from build123d import *

# Parameters (mm, degrees)
BOSS_EXTRUDE1_DEPTH = 3.175


with BuildPart() as part:
    # Sketch1 → Boss-Extrude1 (new body)
    with BuildSketch(Plane.XY):
        with BuildLine():
            Line((0, 0), (0, -1.8034))
            Line((0, -1.8034), (1.778, -6.8834))
            Line((1.778, -6.8834), (1.778, -23.3934))
            Line((1.778, -23.3934), (0, -28.4734))
            Line((0, -28.4734), (0, -33.02))
            Line((0, -33.02), (3.683, -33.02))
            Line((3.683, -33.02), (3.683, -31.369))
            Line((3.683, -31.369), (6.477, -31.369))
            Line((6.477, -31.369), (6.477, -37.719))
            Line((6.477, -37.719), (3.683, -37.719))
            Line((3.683, -37.719), (3.683, -36.068))
            Line((3.683, -36.068), (0, -36.068))
            Line((0, -36.068), (0, -149.521333333))
            Line((0, -149.521333333), (3.683, -149.521333333))
            Line((3.683, -149.521333333), (3.683, -147.870333333))
            Line((3.683, -147.870333333), (6.477, -147.870333333))
            Line((6.477, -147.870333333), (6.477, -154.220333333))
            Line((6.477, -154.220333333), (3.683, -154.220333333))
            Line((3.683, -154.220333333), (3.683, -152.569333333))
            Line((3.683, -152.569333333), (0, -152.569333333))
            Line((0, -152.569333333), (0, -280.162))
            Line((0, -280.162), (3.683, -280.162))
            Line((3.683, -280.162), (3.683, -278.511))
            Line((3.683, -278.511), (6.477, -278.511))
            Line((6.477, -278.511), (6.477, -284.861))
            Line((6.477, -284.861), (3.683, -284.861))
            Line((3.683, -284.861), (3.683, -283.21))
            Line((3.683, -283.21), (0, -283.21))
            Line((0, -283.21), (0, -295.91))
            Line((0, -295.91), (12.7, -295.91))
            Line((12.7, -295.91), (12.7, 0))
            ThreePointArc((12.7, 0), (0, 12.7), (-12.7, 0))
            Line((-12.7, 0), (-3.175, -2.921))
            Line((-3.175, -2.921), (-3.175, 0))
            Line((-3.175, 0), (0, 0))
        make_face()
    extrude(amount=BOSS_EXTRUDE1_DEPTH)


solid = part.part
Verification items for the finished model (mm, model axes). Round coordinates to 2 decimals unless told otherwise and drop trailing zeros. Order: outer loops, then holes, each group sorted by start corner. A loop starts at its lowest first (then second) coordinate and runs counter-clockwise, first axis right, second up.
1. Thickness scan on L1, parallel to Y at x = 3.5, z = 0.7; L2, parallel to X at y = -160, z = 1.15; L3, parallel to X at y = -15, z = 1.95. Record the ranges inside material, lowest first.
Final values:
L1: y = -295.91 to -283.21, -280.16 to -152.57, -149.52 to -36.07, -33.02 to 12.21
L2: x = 0 to 12.7
L3: x = 1.78 to 12.7
2. Go/stop test with flat-tipped pins: P1, Ø0.8, axis at x = 4.5, z = 1, coming from the +Y side; P2, Ø1.5, axis at x = -7, z = 2, coming from the -Y side; P3, Ø0.8, axis at x = 5.5, z = 1, coming from the +Y side. Record where each tip stops, or that it passes through.
Final values:
P1: stops at y = 12.02
P2: stops at y = -1.98
P3: stops at y = 11.63
3. Section check A-A on y = -77.5. Record the cut outline in (x, z) (3 decimals).
Final values:
outline: (0, 0) - (12.7, 0) - (12.7, 3.175) - (0, 3.175) - close
